```python
from build123d import *

# Parameters (mm, degrees)
SKETCH1_W           = 22.86
SKETCH1_H           = 22.86
BOSS_EXTRUDE1_DEPTH = 1.5875
SKETCH2_W           = 9
SKETCH2_H           = 10
BOSS_EXTRUDE2_DEPTH = 10
SKETCH4_W           = 2
SKETCH4_H           = 20
BOSS_EXTRUDE3_DEPTH = 10
SKETCH6_R           = 1.27
CUT_EXTRUDE1_DEPTH  = 20.007624786


with BuildPart() as part:
    # Sketch1 → Boss-Extrude1 (new body)
    with BuildSketch(Plane.XY):
        Rectangle(SKETCH1_W, SKETCH1_H)
    extrude(amount=BOSS_EXTRUDE1_DEPTH)

    # Sketch2 → Boss-Extrude2 (add)
    with BuildSketch(Plane.XY.offset(1.5875)):
        with Locations((-6.93, 0)):
            Rectangle(SKETCH2_W, SKETCH2_H)
    extrude(amount=BOSS_EXTRUDE2_DEPTH)

    # Sketch4 → Boss-Extrude3 (add)
    with BuildSketch(Plane.XY.offset(1.5875)):
        with Locations((10.43, 0)):
            Rectangle(SKETCH4_W, SKETCH4_H)
    extrude(amount=BOSS_EXTRUDE3_DEPTH)

    # Sketch6 → Cut-Extrude1 (cut, through all)
    with BuildSketch(Plane.XY.offset(1.5875)):
        with Locations((-8.89, 8.89)):
            Circle(SKETCH6_R)
        with Locations((-8.89, -8.89)):
            Circle(SKETCH6_R)
    extrude(amount=-CUT_EXTRUDE1_DEPTH, mode=Mode.SUBTRACT)


solid = part.part
```
Work out the finished part from the listing and answer in its coordinate system (mm). A direction names the side the tool comes from. Give positions to 0.01 mm unless a question says otherwise; leave off trailing zeros. Loops run counter-clockwise (first coordinate to the right, second up) from the corner with the lowest first, then second, coordinate; pieces in that order, holes last. Notation, with made-up numbers: (66, 22) -> (99, 22) arc R28 ccw to (99, 51) -> close; hole circle Ø3 at (13, 14). An arc over 180 degrees is marked (long way). Use CSV: the item, a comma, the result in double quotes.
1. Flat-ended cylindrical pins translate along their axes: pin 1 Ø4.5 at (x, z) = (-6, 8.5) entering from +Y; pin 2 Ø2 at (x, z) = (10.5, 4.5) entering from -Y; pin 3 Ø2 at (x, z) = (10.5, 5.5) entering from +Y. Find the tip coordinate at first contact, or state that the pin passes through.
Found:
pin 1,"y = 5"
pin 2,"y = -10"
pin 3,"y = 10"
2. The part is cut by section B-B (z = 3.75). Write down the section's boundary in (x, y).
Found:
outline,"(-11.43, -5) -> (-2.43, -5) -> (-2.43, 5) -> (-11.43, 5) -> close; (9.43, -10) -> (11.43, -10) -> (11.43, 10) -> (9.43, 10) -> close"
3. The part is cut by section A-A (y = -8.89). Write down the section's boundary in (x, z), then the cut area to 3 significant figures.
Found:
outline,"(-11.43, 0) -> (-10.16, 0) -> (-10.16, 1.59) -> (-11.43, 1.59) -> close; (-7.62, 0) -> (11.43, 0) -> (11.43, 11.59) -> (9.43, 11.59) -> (9.43, 1.59) -> (-7.62, 1.59) -> close"
area,"52.3 mm^2"
4. The mould has two halves that part along X. Classify faces 1 (the flat face through (11.43, 0, 6)), 2 (the flat face through (-7, 5, 7)), 3 (the flat face through (0, 0, 1.588)): +X half, -X half, draft (parallel to the pull), parting line (faces both ways), or undercut.
Found:
face 1,"+X half"
face 2,"draft"
face 3,"undercut"
5. A tool of negligible diameter and unlimited length cuts with its end or side. For faces 4 (the flat face through (10, 10, 7)), 5 (the flat face through (-7, -5, 7)), 6 (the flat face through (10, -10, 7)), 7 (the flat face through (-2.43, 0, 7)), from which of +Z, -Z, +X, -X, +Y, -Y can it reach the whole face along a straight path? Write none if from no direction.
Found:
face 4,"+Z, +X, -X, +Y"
face 5,"+Z, -X, -Y"
face 6,"+Z, +X, -X, -Y"
face 7,"+Z, +Y, -Y"
6. Straight lines are drawn through the part: line 1 (Y direction, x = -8.89, z = 0.45); line 2 (X direction, y = 2, z = 2.75); line 3 (Y direction, x = -7.5, z = 6.75). For each, find the intervals that lie inside material, in ascending order.
Found:
line 1,"-11.43 to -10.16, -7.62 to 7.62, 10.16 to 11.43"
line 2,"-11.43 to -2.43, 9.43 to 11.43"
line 3,"-5 to 5"
7. The part is cut by section C-C (x = -8.89). Write down the section's boundary in (y, z).
Found:
outline,"(-11.43, 0) -> (-10.16, 0) -> (-10.16, 1.59) -> (-11.43, 1.59) -> close; (-7.62, 0) -> (7.62, 0) -> (7.62, 1.59) -> (5, 1.59) -> (5, 11.59) -> (-5, 11.59) -> (-5, 1.59) -> (-7.62, 1.59) -> close; (10.16, 0) -> (11.43, 0) -> (11.43, 1.59) -> (10.16, 1.59) -> close"
8. The part is cut by section D-D (y = -2.5). Write down the section's boundary in (x, z).
Found:
outline,"(-11.43, 0) -> (11.43, 0) -> (11.43, 11.59) -> (9.43, 11.59) -> (9.43, 1.59) -> (-2.43, 1.59) -> (-2.43, 11.59) -> (-11.43, 11.59) -> close"
